Work out the finished part from the listing and answer in its coordinate system (mm). A direction names the side the tool comes from. Coordinates: 2 decimals unless noted, no trailing zeros. Loops run counter-clockwise (first coordinate to the right, second up) from the corner with the lowest first, then second, coordinate; pieces in that order, holes last. Notation, with made-up numbers: (73.25, -26.75) - (102.25, -26.75) arc R8 cw to (102.25, -20.75) - close; hole circle Ø5 at (68.5, 89). An arc over 180 degrees is marked (long way). Write each question's results on one line, items separated by ' | '. Start each with the question number.
1. A cutting plane is placed at A-A on z = 2.5. Determine the outline of the cut face in (x, y).
2. A cutting plane is placed at D-D on x = 20.5. Determine the outline of the cut face in (y, z), then the cut area to 3 significant figures.
3. A cutting plane is placed at B-B on x = -25.5. Determine the outline of the cut face in (y, z).
4. Which of the six approach directions +Z, -Z, +X, -X, +Y, -Y give full straight-line access (tool end or side, diameter ignored) to faces 1 (the flat face through (-8, 0, 4)), 2 (the cylindrical face through (1.79, 1.48, -0.75))?
5. Find the intervals of material crossed by line 1 along X through (y, z) = (2.1, -7); line 2 along Z through (x, y) = (-5, 0.5); line 3 along Z through (x, y) = (21, 0.4), in increasing order. Write a range as [from, to].
6. A cutting plane is placed at C-C on z = 7.75. Determine the outline of the cut face in (x, y).
7. Each of these flat-tipped pins is pushed along its axis until it touches: P1, Ø1.5, axis at y = 2, z = -17.5, coming from the +X side; P2, Ø1.5, axis at x = 0, y = 1.5, coming from the -Z side. Where does it stop, or does it pass through?
8. Determine the mould class of faces 3 (the flat face through (-17.5, 1, -15)), 4 (the flat face through (-25, 1, -20)), 5 (the cylindrical face through (-4.9, 1.5, 18.5)) for opening direction X: released by +X, released by -X, zero draft, split by the parting line, or undercut.
from build123d import *

# Parameters (mm, degrees)
SKETCH_1_W          = 65
SKETCH_1_H          = 40
EXTRUDE_1_DEPTH     = 3
SKETCH_2_R          = 1.55
CUT_EXTRUDE_1_DEPTH = 10
SKETCH_3_W          = 50
SKETCH_3_H          = 10
CUT_EXTRUDE_2_DEPTH = 10
SKETCH_4_W          = 24
SKETCH_4_H          = 14
CUT_EXTRUDE_3_DEPTH = 10
SKETCH_5_R          = 1.1
CUT_EXTRUDE_4_DEPTH = 10
SKETCH_6_R          = 1.5
CUT_EXTRUDE_5_DEPTH = 25
HOLE_WIZARD_1_D     = 3


with BuildPart() as part:
    # 草图1 → 凸台-拉伸1 (new body)
    with BuildSketch(Plane(origin=(0, 0, 0), x_dir=(1, 0, 0), z_dir=(0, 1, 0))):
        Rectangle(SKETCH_1_W, SKETCH_1_H)
    extrude(amount=EXTRUDE_1_DEPTH)

    # 草图2 → 切除-拉伸1 (cut)
    with BuildSketch(Plane(origin=(0, 0, 0), x_dir=(-1, 0, 0), z_dir=(0, -1, 0))):
        with Locations(Location((25.5, -15, 0), (0, 0, 90))):
            Circle(SKETCH_2_R)
        with Locations(Location((25.5, 5, 0), (0, 0, 90))):
            Circle(SKETCH_2_R)
    extrude(amount=-CUT_EXTRUDE_1_DEPTH, mode=Mode.SUBTRACT)

    # 草图3 → 切除-拉伸2 (cut)
    with BuildSketch(Plane(origin=(0, 0, 0), x_dir=(-1, 0, 0), z_dir=(0, -1, 0))):
        with Locations((-7.5, 15)):
            Rectangle(SKETCH_3_W, SKETCH_3_H)
    extrude(amount=-CUT_EXTRUDE_2_DEPTH, mode=Mode.SUBTRACT)

    # 草图4 → 切除-拉伸3 (cut)
    with BuildSketch(Plane(origin=(0, 0, 0), x_dir=(-1, 0, 0), z_dir=(0, -1, 0))):
        with Locations((-12.32495, -7.75)):
            Rectangle(SKETCH_4_W, SKETCH_4_H)
    extrude(amount=-CUT_EXTRUDE_3_DEPTH, mode=Mode.SUBTRACT)

    # 草图5 → 切除-拉伸4 (cut)
    with BuildSketch(Plane(origin=(0, 3, 0), x_dir=(1, 0, 0), z_dir=(0, 1, 0))):
        with Locations(Location((26.17495, -7.75, 0), (0, 0, 270))):
            Circle(SKETCH_5_R)
        with Locations(Location((-1.52505, -7.75, 0), (0, 0, 270))):
            Circle(SKETCH_5_R)
    extrude(amount=-CUT_EXTRUDE_4_DEPTH, mode=Mode.SUBTRACT)

    # 草图6 → 切除-拉伸5 (cut)
    with BuildSketch(Plane(origin=(0, 0, 0), x_dir=(-1, 0, 0), z_dir=(0, -1, 0))):
        with Locations(Location((-15.074975, -17, 0), (0, 0, 90))):
            Circle(SKETCH_6_R)
        with Locations(Location((4.925025, -17, 0), (0, 0, 90))):
            Circle(SKETCH_6_R)
        with Locations(Location((-15.074975, 7, 0), (0, 0, 90))):
            Circle(SKETCH_6_R)
        with Locations(Location((4.925025, 7, 0), (0, 0, 90))):
            Circle(SKETCH_6_R)
    extrude(amount=-CUT_EXTRUDE_5_DEPTH, mode=Mode.SUBTRACT)

    # 孔1 (through all)
    with Locations(Plane(origin=(0, 3, 0), x_dir=(1, 0, 0), z_dir=(0, 1, 0))):
        with Locations((-16, 10), (1.82495, -0.75), (22.82495, -0.75), (22.82495, -14.75), (1.82495, -14.75)):
            Hole(HOLE_WIZARD_1_D / 2)


solid = part.part
Values:
1) outline: (-32.5, 0) - (0.32, 0) - (0.32, 3) - (-32.5, 3) - close; (24.32, 0) - (32.5, 0) - (32.5, 3) - (24.32, 3) - close
2) outline: (0, -10) - (3, -10) - (3, 0.75) - (0, 0.75) - close; (0, 14.75) - (3, 14.75) - (3, 20) - (0, 20) - close | area: 48.0 mm^2
3) outline: (0, -20) - (3, -20) - (3, -6.55) - (0, -6.55) - close; (0, -3.45) - (3, -3.45) - (3, 13.45) - (0, 13.45) - close; (0, 16.55) - (3, 16.55) - (3, 20) - (0, 20) - close
4) face 1: +Z, -Z, +X, -X, -Y | face 2: +Y, -Y
5) line 1: [-32.5, -6.43], [-3.43, 13.57], [16.57, 32.5] | line 2: [-10, -8.5], [-5.5, 15.5], [18.5, 20] | line 3: [-10, 0.75], [14.75, 20]
6) outline: (-32.5, 0) - (-2.63, 0) - (-2.63, 3) - (-32.5, 3) - close; (-0.43, 0) - (0.32, 0) - (0.32, 3) - (-0.43, 3) - close; (24.32, 0) - (25.07, 0) - (25.07, 3) - (24.32, 3) - close; (27.27, 0) - (32.5, 0) - (32.5, 3) - (27.27, 3) - close
7) P1: x = -17.5 | P2: z = -10
8) face 3: released by +X | face 4: zero draft | face 5: undercut
